from build123d import *

# Parameters (mm, degrees)
CROQUIS1_R              = 10.4
SALIENTE_EXTRUIR1_DEPTH = 2.4
SALIENTE_EXTRUIR2_START = -2.4
CROQUIS2_R              = 4.4
SALIENTE_EXTRUIR2_DEPTH = 5.5
CROQUIS3_R              = 3
CORTAR_EXTRUIR1_DEPTH   = 2.8
CROQUIS4_R              = 0.75
CORTAR_EXTRUIR2_DEPTH   = 16.030968033
CROQUIS5_R              = 1.5
CORTAR_EXTRUIR3_DEPTH   = 15.971973818


with BuildPart() as part:
    # Croquis1 → Saliente-Extruir1 (new body)
    with BuildSketch(Plane(origin=(0, 0, 0), x_dir=(1, 0, 0), z_dir=(0, 1, 0))):
        with Locations(Location((0, 0, 0), (0, 0, 270))):
            Circle(CROQUIS1_R)
    extrude(amount=SALIENTE_EXTRUIR1_DEPTH)

    # Croquis2 → Saliente-Extruir2 (add)
    with BuildSketch(Plane(origin=(0, 2.4, 0), x_dir=(1, 0, 0), z_dir=(0, 1, 0)).offset(SALIENTE_EXTRUIR2_START)):
        with Locations(Location((0, 0, 0), (0, 0, 270))):
            Circle(CROQUIS2_R)
    extrude(amount=SALIENTE_EXTRUIR2_DEPTH)

    # Croquis3 → Cortar-Extruir1 (cut)
    with BuildSketch(Plane(origin=(0, 5.5, 0), x_dir=(1, 0, 0), z_dir=(0, 1, 0))):
        with Locations(Location((0, 0, 0), (0, 0, 270))):
            Circle(CROQUIS3_R)
    extrude(amount=-CORTAR_EXTRUIR1_DEPTH, mode=Mode.SUBTRACT)

    # Croquis4 → Cortar-Extruir2 (cut, through all)
    with BuildSketch(Plane(origin=(0, 2.4, 0), x_dir=(1, 0, 0), z_dir=(0, 1, 0))):
        with Locations(Location((0, 7.875, 0), (0, 0, 270))):
            Circle(CROQUIS4_R)
        with Locations(Location((7.875, 0, 0), (0, 0, 270))):
            Circle(CROQUIS4_R)
        with Locations(Location((0, -7.875, 0), (0, 0, 270))):
            Circle(CROQUIS4_R)
        with Locations(Location((-7.875, 0, 0), (0, 0, 270))):
            Circle(CROQUIS4_R)
    extrude(amount=-CORTAR_EXTRUIR2_DEPTH, mode=Mode.SUBTRACT)

    # Croquis5 → Cortar-Extruir3 (cut, through all)
    with BuildSketch(Plane(origin=(0, 2.7, 0), x_dir=(1, 0, 0), z_dir=(0, 1, 0))):
        with Locations(Location((0, 0, 0), (0, 0, 270))):
            Circle(CROQUIS5_R)
    extrude(amount=-CORTAR_EXTRUIR3_DEPTH, mode=Mode.SUBTRACT)


solid = part.part
Work out the finished part from the listing and answer in its coordinate system (mm). A direction names the side the tool comes from. Give positions to 0.01 mm unless a question says otherwise; leave off trailing zeros. Write each loop counter-clockwise with the first axis right and the second up, starting at its lowest first coordinate (ties: lowest second). Pieces come first, ordered by that corner, then holes.
Q1. The part is cut by section C-C on y = 3.15. Give the vertices of the cut face in (x, z).
Answer:
outline: circle Ø8.8 at (0, 0); hole circle Ø6 at (0, 0)
Q2. Straight lines are drawn through the part: L1, parallel to X at y = 1.25, z = 0 (3 decimals); L2, parallel to X at y = 4.7, z = 0; L3, parallel to Y at x = 6, z = -5.25. For each, find the intervals that lie inside material, in ascending order.
Answer:
L1: x = -10.4 to -8.625, -7.125 to -1.5, 1.5 to 7.125, 8.625 to 10.4
L2: x = -4.4 to -3, 3 to 4.4
L3: y = 0 to 2.4
Q3. A tool of negligible diameter and unlimited length cuts with its end or side. For faces 1 (the face through (-1.3, 2.7, 1.3)), 2 (the face through (-7.65, 1.217, 0.715)), from which of +Z, -Z, +X, -X, +Y, -Y can it reach the whole face along a straight path? Write none if from no direction.
Answer:
face 1: +Y
face 2: +Y, -Y
Q4. Given pin 1 (1.5 mm diameter, centred on x = 3.5, y = 5, fed in from -Z); pin 2 (1 mm diameter, centred on y = 1.5, z = -6, fed in from -X), each flat-ended and moving along its own axis, determine where each tip first touches the part or whether it passes through.
Answer:
pin 1: stops at z = -3.43
pin 2: stops at x = -8.83
Q5. For a pull along Z with two mould halves and no side action, classify faces 3 (the face through (0.45, 1.37, 1.43)), 4 (the face through (-3, 5.5, 1)), 5 (the face through (4.363, 3.928, -0.573)) as released by +Z, released by -Z, zero draft, split by the parting line, or undercut.
Answer:
face 3: undercut
face 4: zero draft
face 5: split by the parting line
Q6. The part is cut by section B-B on x = 0. Give the vertices of the cut face in (y, z) (3 decimals), and give its area (3 significant figures).
Answer:
outline: (0, -10.4) - (2.4, -10.4) - (2.4, -8.625) - (0, -8.625) - close; (0, -7.125) - (2.4, -7.125) - (2.4, -4.4) - (5.5, -4.4) - (5.5, -3) - (2.7, -3) - (2.7, -1.5) - (0, -1.5) - close; (0, 1.5) - (2.7, 1.5) - (2.7, 3) - (5.5, 3) - (5.5, 4.4) - (2.4, 4.4) - (2.4, 7.125) - (0, 7.125) - close; (0, 8.625) - (2.4, 8.625) - (2.4, 10.4) - (0, 10.4) - close
area: 45.1 mm2
Q7. The part is cut by section A-A on z = 0. Give the vertices of the cut face in (x, y) (3 decimals), and give its area (3 significant figures).
Answer:
outline: (-10.4, 0) - (-8.625, 0) - (-8.625, 2.4) - (-10.4, 2.4) - close; (-7.125, 0) - (-1.5, 0) - (-1.5, 2.7) - (-3, 2.7) - (-3, 5.5) - (-4.4, 5.5) - (-4.4, 2.4) - (-7.125, 2.4) - close; (1.5, 0) - (7.125, 0) - (7.125, 2.4) - (4.4, 2.4) - (4.4, 5.5) - (3, 5.5) - (3, 2.7) - (1.5, 2.7) - close; (8.625, 0) - (10.4, 0) - (10.4, 2.4) - (8.625, 2.4) - close
area: 45.1 mm2
Q8. The part is cut by section D-D on z = 3.25. Give the vertices of the cut face in (x, y), and give its area (3 significant figures).
Answer:
outline: (-9.88, 0) - (9.88, 0) - (9.88, 2.4) - (2.97, 2.4) - (2.97, 5.5) - (-2.97, 5.5) - (-2.97, 2.4) - (-9.88, 2.4) - close
area: 65.8 mm2
